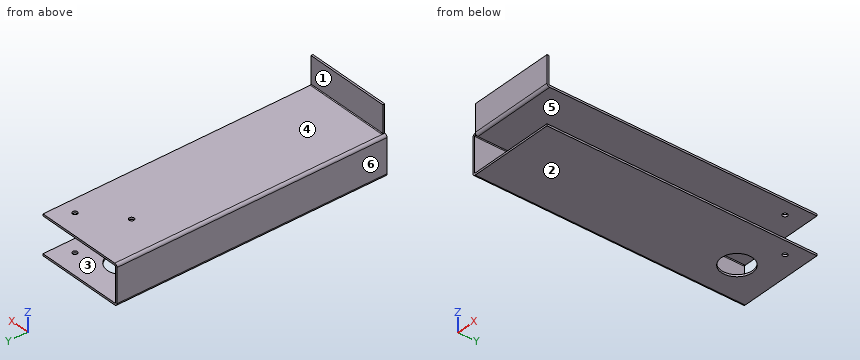
from build123d import *

# Parameters (mm, degrees)
SKETCH1_W                    = 90
SKETCH1_H                    = 275
BASE_FLANGE1_DEPTH           = 2
EDGE_FLANGE1_STRIP_W         = 9.4732
EDGE_FLANGE1_STRIP_H         = 2
EDGE_FLANGE1_STRIP_CUT_DEPTH = 275
EDGE_FLANGE1_DEPTH           = 275
EDGE_FLANGE2_STRIP_W         = 9.4732
EDGE_FLANGE2_STRIP_H         = 2
EDGE_FLANGE2_STRIP_CUT_DEPTH = 275
EDGE_FLANGE2_DEPTH           = 275
EDGE_FLANGE3_STRIP_W         = 9.4732
EDGE_FLANGE3_STRIP_H         = 2
EDGE_FLANGE3_STRIP_CUT_DEPTH = 87.2634
EDGE_FLANGE3_DEPTH           = 87.2634
CUT_EXTRUDE2_REACH           = 294.104
SKETCH18_R                   = 2.5
CUT_EXTRUDE1_REACH           = 299.236
SKETCH17_R                   = 15.875
SKETCH17_R_2                 = 2.5


# Sheet-metal steps are written as plain solids
with BuildPart() as part:
    # Sketch1 → Base-Flange1 (new body)
    with BuildSketch(Plane.XY):
        with Locations((45, 137.5)):
            Rectangle(SKETCH1_W, SKETCH1_H)
    extrude(amount=-BASE_FLANGE1_DEPTH)

    # Edge-Flange1 strip (across the edge) → Edge-Flange1 strip cut (cut)
    with BuildSketch(Plane(origin=(0, 0, -2), x_dir=(1, 0, 0), z_dir=(0, 1, 0))):
        with Locations((-2, -1)):
            Rectangle(EDGE_FLANGE1_STRIP_W, EDGE_FLANGE1_STRIP_H)
    extrude(amount=EDGE_FLANGE1_STRIP_CUT_DEPTH, mode=Mode.SUBTRACT)

    # Edge-Flange1 section (across the edge) → Edge-Flange1 (add)
    with BuildSketch(Plane(origin=(0, 0, -2), x_dir=(1, 0, 0), z_dir=(0, 1, 0))):
        with BuildLine():
            Line((0, 0.7366), (0, 38))
            Line((0, 38), (2, 38))
            Line((2, 38), (2, 0.7366))
            ThreePointArc((2, 0.7366), (2.215745145, 0.215745145), (2.7366, 0))
            Line((2.7366, 0), (2.7366, -2))
            ThreePointArc((2.7366, -2), (0.801531583, -1.198468417), (0, 0.7366))
        make_face()
    extrude(amount=EDGE_FLANGE1_DEPTH)

    # Edge-Flange2 strip (across the edge) → Edge-Flange2 strip cut (cut)
    with BuildSketch(Plane(origin=(2, 0, -40), x_dir=(0, 0, 1), z_dir=(0, 1, 0))):
        with Locations((-2, -1)):
            Rectangle(EDGE_FLANGE2_STRIP_W, EDGE_FLANGE2_STRIP_H)
    extrude(amount=EDGE_FLANGE2_STRIP_CUT_DEPTH, mode=Mode.SUBTRACT)

    # Edge-Flange2 section (across the edge) → Edge-Flange2 (add)
    with BuildSketch(Plane(origin=(2, 0, -40), x_dir=(0, 0, 1), z_dir=(0, 1, 0))):
        with BuildLine():
            Line((0, 0.7366), (0, 88))
            Line((0, 88), (2, 88))
            Line((2, 88), (2, 0.7366))
            ThreePointArc((2, 0.7366), (2.215745145, 0.215745145), (2.7366, 0))
            Line((2.7366, 0), (2.7366, -2))
            ThreePointArc((2.7366, -2), (0.801531583, -1.198468417), (0, 0.7366))
        make_face()
    extrude(amount=EDGE_FLANGE2_DEPTH)

    # Edge-Flange3 strip (across the edge) → Edge-Flange3 strip cut (cut)
    with BuildSketch(Plane.YZ.offset(2.7366)):
        with Locations((-2, -1)):
            Rectangle(EDGE_FLANGE3_STRIP_W, EDGE_FLANGE3_STRIP_H)
    extrude(amount=EDGE_FLANGE3_STRIP_CUT_DEPTH, mode=Mode.SUBTRACT)

    # Edge-Flange3 section (across the edge) → Edge-Flange3 (add)
    with BuildSketch(Plane.YZ.offset(2.7366)):
        with BuildLine():
            Line((0, 0.7366), (0, 28))
            Line((0, 28), (2, 28))
            Line((2, 28), (2, 0.7366))
            ThreePointArc((2, 0.7366), (2.215745145, 0.215745145), (2.7366, 0))
            Line((2.7366, 0), (2.7366, -2))
            ThreePointArc((2.7366, -2), (0.801531583, -1.198468417), (0, 0.7366))
        make_face()
    extrude(amount=EDGE_FLANGE3_DEPTH)

    # Sketch18 → Cut-Extrude2 (cut, up to next)
    with BuildSketch(Plane.XY, mode=Mode.PRIVATE) as cut_extrude2_sk1:
        with Locations((40.19, 226.48)):
            Circle(SKETCH18_R)
    cut_extrude2_tool1 = extrude(cut_extrude2_sk1.sketch, amount=-CUT_EXTRUDE2_REACH, mode=Mode.PRIVATE) & part.part
    # Sketch18 → Cut-Extrude2 (cut, up to next)
    with BuildSketch(Plane.XY, mode=Mode.PRIVATE) as cut_extrude2_sk2:
        with Locations((75, 255)):
            Circle(SKETCH18_R)
    cut_extrude2_tool2 = extrude(cut_extrude2_sk2.sketch, amount=-CUT_EXTRUDE2_REACH, mode=Mode.PRIVATE) & part.part
    add(cut_extrude2_tool1.solids().sort_by_distance((40.19, 226.48, 0))[0], mode=Mode.SUBTRACT)
    add(cut_extrude2_tool2.solids().sort_by_distance((75, 255, 0))[0], mode=Mode.SUBTRACT)

    # Sketch17 → Cut-Extrude1 (cut, up to next)
    with BuildSketch(Plane(origin=(0, 0, -40), x_dir=(-1, 0, 0), z_dir=(0, 0, -1)), mode=Mode.PRIVATE) as cut_extrude1_sk1:
        with Locations((-40.1866, 235.2)):
            Circle(SKETCH17_R)
    cut_extrude1_tool1 = extrude(cut_extrude1_sk1.sketch, amount=-CUT_EXTRUDE1_REACH, mode=Mode.PRIVATE) & part.part
    # Sketch17 → Cut-Extrude1 (cut, up to next)
    with BuildSketch(Plane(origin=(0, 0, -40), x_dir=(-1, 0, 0), z_dir=(0, 0, -1)), mode=Mode.PRIVATE) as cut_extrude1_sk2:
        with Locations(Location((-75, 255, 0), (0, 0, 180))):
            Circle(SKETCH17_R_2)
    cut_extrude1_tool2 = extrude(cut_extrude1_sk2.sketch, amount=-CUT_EXTRUDE1_REACH, mode=Mode.PRIVATE) & part.part
    add(cut_extrude1_tool1.solids().sort_by_distance((40.1866, 235.2, -40))[0], mode=Mode.SUBTRACT)
    add(cut_extrude1_tool2.solids().sort_by_distance((75, 255, -40))[0], mode=Mode.SUBTRACT)


solid = part.part
Work out the finished part from the listing and answer in its coordinate system (mm). Face numbers are marked on the shaded views. A direction names the side the tool comes from. Give positions to 0.01 mm unless a question says otherwise; leave off trailing zeros. Loops run counter-clockwise (first coordinate to the right, second up) from the corner with the lowest first, then second, coordinate; pieces in that order, holes last. Notation, with made-up numbers: (20, 14) -> (62, 14) arc R18 cw to (62, 22) -> close; hole circle Ø9 at (35, 39). An arc over 180 degrees is marked (long way). Use a Markdown table: item, result. Add a question column.
1) Consider line 1 along Z through (x, y) = (51, 131.5); line 2 along Y through (x, z) = (75, -39.25); line 3 along Y through (x, z) = (40.19, -1.15). Determine where each line is inside the solid, lowest interval first.
2) The part is cut by section B-B, the plane y = 255. Determine the outline of the cut face in (x, z).
3) Which of the six approach directions +Z, -Z, +X, -X, +Y, -Y give full straight-line access (tool end or side, diameter ignored) to the marked faces 1, 2 and 3?
4) Each of these flat-tipped pins is pushed along its axis until it touches: P1, Ø13.5, axis at x = 42.5, z = 19.5, coming from the +Y side; P2, Ø17.5, axis at y = 183.5, z = -15, coming from the +X side; P3, Ø3, axis at x = 40.19, y = 226.48, coming from the +Z side; P4, Ø6, axis at x = 29, y = 58.5, coming from the +Z side. Where does it stop, or does it pass through?
5) The part is cut by section D-D, the plane x = 40.19. Determine the outline of the cut face in (y, z) (3 decimals), plus the area to 3 significant figures.
6) The part is cut by section C-C, the plane x = 60.5. Determine the outline of the cut face in (y, z), plus the area to 3 significant figures.
7) The part is cut by section A-A, the plane x = 75. Determine the outline of the cut face in (y, z), plus the area to 3 significant figures.
8) For a pull along Z with two mould halves and no side action, classify the marked faces 4, 5 and 6 as +Z half, -Z half, draft (parallel to the pull), parting line (faces both ways), or undercut.
Reported:
| question | item | result |
|---|---|---|
| 1 | line 1 | z = -40 to -38, -2 to 0 |
| 1 | line 2 | y = 0 to 252.5, 257.5 to 275 |
| 1 | line 3 | y = 0.75 to 223.98, 228.98 to 275 |
| 2 | outline | (0, -37.26) arc R2.74 ccw to (2.74, -40) -> (72.5, -40) -> (72.5, -38) -> (2.74, -38) arc R0.74 cw to (2, -37.26) -> (2, -2.74) arc R0.74 cw to (2.74, -2) -> (72.5, -2) -> (72.5, 0) -> (2.74, 0) arc R2.74 ccw to (0, -2.74) -> close; (77.5, -40) -> (90, -40) -> (90, -38) -> (77.5, -38) -> close; (77.5, -2) -> (90, -2) -> (90, 0) -> (77.5, 0) -> close |
| 3 | face 1 | +Z, +X, -X, +Y |
| 3 | face 2 | -Z, +X, -X, +Y, -Y |
| 3 | face 3 | +X, +Y, -Y |
| 4 | P1 | stops at y = 2 |
| 4 | P2 | stops at x = 2 |
| 4 | P3 | passes through |
| 4 | P4 | stops at z = 0 |
| 5 | outline | (0, -40) -> (219.325, -40) -> (219.325, -38) -> (0, -38) -> close; (0, 0.737) arc R2.737 ccw to (2.737, -2) -> (223.98, -2) -> (223.98, 0) -> (2.737, 0) arc R0.737 cw to (2, 0.737) -> (2, 28) -> (0, 28) -> close; (228.98, -2) -> (275, -2) -> (275, 0) -> (228.98, 0) -> close; (251.075, -40) -> (275, -40) -> (275, -38) -> (251.075, -38) -> close |
| 5 | area | 1,080 mm^2 |
| 6 | outline | (0, -40) -> (275, -40) -> (275, -38) -> (0, -38) -> close; (0, 0.74) arc R2.74 ccw to (2.74, -2) -> (275, -2) -> (275, 0) -> (2.74, 0) arc R0.74 cw to (2, 0.74) -> (2, 28) -> (0, 28) -> close |
| 6 | area | 1,150 mm^2 |
| 7 | outline | (0, -40) -> (252.5, -40) -> (252.5, -38) -> (0, -38) -> close; (0, 0.74) arc R2.74 ccw to (2.74, -2) -> (252.5, -2) -> (252.5, 0) -> (2.74, 0) arc R0.74 cw to (2, 0.74) -> (2, 28) -> (0, 28) -> close; (257.5, -40) -> (275, -40) -> (275, -38) -> (257.5, -38) -> close; (257.5, -2) -> (275, -2) -> (275, 0) -> (257.5, 0) -> close |
| 7 | area | 1,130 mm^2 |
| 8 | face 4 | +Z half |
| 8 | face 5 | undercut |
| 8 | face 6 | draft |
